For this review, use the dimensioned drawing (mm, ordinates from the lowest corner) and the shaded views. Coordinates: 2 decimals unless noted, no trailing zeros. Order: outer loops, then holes, each group sorted by start corner. A loop starts at its lowest first (then second) coordinate and runs counter-clockwise, first axis right, second up. Notation, with made-up numbers: M 59.25,70 L 93.25,70 A31 ccw 93.25,108 Z; hole C -22,51.25 d7. An arc over 180 degrees is marked long. Answer as CSV lines item,"result". Start each with the question number.
Q1. Consider section D-D on z = 5.5. Write out the cut boundary in (x, y), and give its area (3 significant figures).
Q2. Consider section A-A on x = 24. Write out the cut boundary in (y, z) (3 decimals).
Q3. Wall thickness on L1, parallel to X at y = 36.5, z = 3.25; L2, parallel to Y at x = 12.5, z = 12; L3, parallel to Z at x = 10.5, y = 15.5 (3 decimals): over which ranges is each line inside the solid? List them lowest first. Write a range as [from, to].
Q4. Consider section C-C on y = 17. Write out the cut boundary in (x, z) (3 decimals), and give its area (3 significant figures).
Q5. For P1, Ø20.5, axis at x = 21, y = 185.5, coming from the +Z side (3 decimals); P2, Ø1, axis at x = 7.5, y = 88, coming from the +Z side; P3, Ø1, axis at x = 10.5, z = 17.5, coming from the +Y side, all flat-tipped, find the tip position at first contact; note any pin that passes through.
Q6. Consider section B-B on y = 164. Write out the cut boundary in (x, z) (3 decimals), and give its area (3 significant figures).
Q7. The part is to be moulded in two halves that separate along X. For the marked faces 1, 2 and 3, say which applies: +X half, -X half, draft (parallel to the pull), parting line (faces both ways), or undercut.
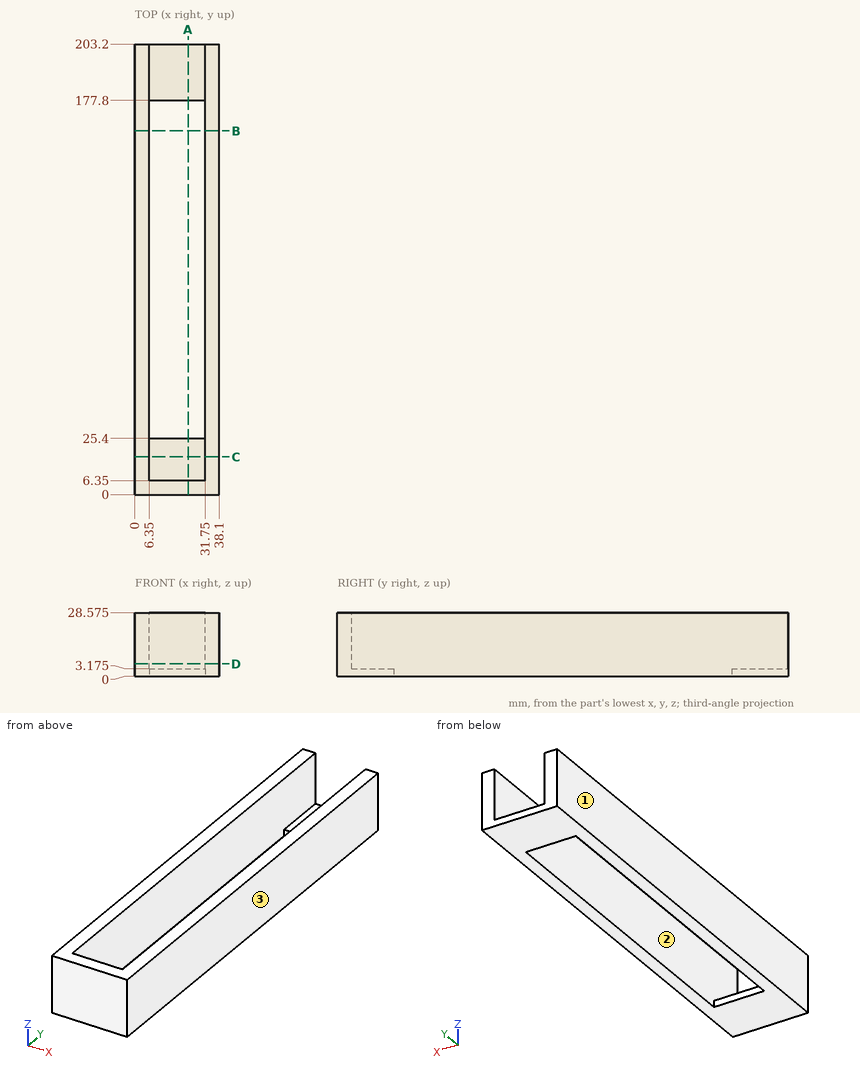
Evaluation:
1,outline,"M 0,0 L 38.1,0 L 38.1,203.2 L 31.75,203.2 L 31.75,6.35 L 6.35,6.35 L 6.35,203.2 L 0,203.2 Z"
1,area,"2,740 mm²"
2,outline,"M 0,0 L 25.4,0 L 25.4,3.175 L 6.35,3.175 L 6.35,28.575 L 0,28.575 Z; M 177.8,0 L 203.2,0 L 203.2,3.175 L 177.8,3.175 Z"
3,L1,"x = [0, 6.35], [31.75, 38.1]"
3,L2,"y = [0, 6.35]"
3,L3,"z = [0, 3.175]"
4,outline,"M 0,0 L 38.1,0 L 38.1,28.575 L 31.75,28.575 L 31.75,3.175 L 6.35,3.175 L 6.35,28.575 L 0,28.575 Z"
4,area,"444 mm²"
5,P1,"stops at z = 3.175"
5,P2,"passes through"
5,P3,"stops at y = 6.35"
6,outline,"M 0,0 L 6.35,0 L 6.35,28.575 L 0,28.575 Z; M 31.75,0 L 38.1,0 L 38.1,28.575 L 31.75,28.575 Z"
6,area,"363 mm²"
7,face 1,"-X half"
7,face 2,"undercut"
7,face 3,"+X half"
